Geometry: final body of the model. Coordinates: model frame, mm. A direction names the side the tool comes from. Round coordinates to 2 decimals unless told otherwise and drop trailing zeros. Order: outer loops, then holes, each group sorted by start corner. A loop starts at its lowest first (then second) coordinate and runs counter-clockwise, first axis right, second up. Notation, with made-up numbers: M 6,81 L 64,81 A17 ccw 64,96 Z; hole C 38.5,46.5 d1. An arc over 180 degrees is marked long. Return JSON: item names as keys, results as strings. Group by question number.
Q1. Cut plane B-B on x = 0. Output: boundary loops of the cut face in (y, z), and give its area (3 significant figures).
Q2. Cut plane A-A on y = 4.25. Output: boundary loops of the cut face in (x, z).
Q3. Access query for faces 1 (the face through (-1.5, 2.46, 0.07)), 2 (the face through (-1.74, 3.94, 0.99)), 3 (the face through (2, 8, 0)). Directions: +Z, -Z, +X, -X, +Y, -Y. A direction counts if a zero-diameter tool reaches every point of the face in a straight line with its end or side. Return the directions, or none.
Q4. Contact query for flat-ended pins moving along their axis: pin 1 (1.5 mm diameter, centred on x = 1, y = 10.5, fed in from -Z); pin 2 (1.8 mm diameter, centred on x = 0, z = 0, fed in from -Y); pin 3 (1.5 mm diameter, centred on y = 11.5, z = 1, fed in from +X). Output: stop coordinate, or through.
Q5. Mould query, pull axis Z, two halves, no side actions, for faces 4 (the face through (0, 16, 0)), 5 (the face through (0, 5, 0)), 6 (the face through (-1.5, 11.94, -0.07)). Classes: released by +Z, released by -Z, zero draft, split by the parting line, or undercut.
Q6. Ray query, probe 1 along Z at (x, y) = (0, 1.4); probe 2 along Y at (x, z) = (-1.4, 1.1); probe 3 along Y at (x, z) = (0.05, -0.5). Return the intervals inside material, ascending.
Q7. Cut plane C-C on z = 1. Output: boundary loops of the cut face in (x, y).
Q8. Cut plane D-D on y = 6. Output: boundary loops of the cut face in (x, z).
```python
from build123d import *

# Parameters (mm, degrees)
EXTRUDE_1_DEPTH     = 8
SKETCH_2_R          = 1.5
EXTRUDE_2_DEPTH     = 8
SKETCH_3_R          = 1.5
CUT_EXTRUDE_1_DEPTH = 5


with BuildPart() as part:
    # 草图1 → 凸台-拉伸1 (new body)
    with BuildSketch(Plane(origin=(0, 0, 0), x_dir=(1, 0, 0), z_dir=(0, 1, 0))):
        Polygon((-1.154700538, -2), (1.154700538, -2), (2.309401077, 0), (1.154700538, 2), (-1.154700538, 2), (-2.309401077, 0), align=None)
    extrude(amount=EXTRUDE_1_DEPTH)

    # 草图2 → 凸台-拉伸2 (add)
    with BuildSketch(Plane(origin=(0, 8, 0), x_dir=(1, 0, 0), z_dir=(0, 1, 0))):
        Circle(SKETCH_2_R)
    extrude(amount=EXTRUDE_2_DEPTH)

    # 草图3 → 切除-拉伸1 (cut)
    with BuildSketch(Plane.XZ):
        Circle(SKETCH_3_R)
    extrude(amount=-CUT_EXTRUDE_1_DEPTH, mode=Mode.SUBTRACT)


solid = part.part
```
Result sheet:
{
 "1": {"outline": "M 0,-2 L 8,-2 L 8,-1.5 L 16,-1.5 L 16,1.5 L 8,1.5 L 8,2 L 0,2 L 0,1.5 L 5,1.5 L 5,-1.5 L 0,-1.5 Z", "area": "41.0 mm²"},
 "2": {"outline": "M -2.31,0 L -1.15,-2 L 1.15,-2 L 2.31,0 L 1.15,2 L -1.15,2 Z; hole C 0,0 d3"},
 "3": {"face 1": "-Y", "face 2": "+Z, -X, +Y, -Y", "face 3": "+Y"},
 "4": {"pin 1": "stops at z = -1.48", "pin 2": "stops at y = 5", "pin 3": "stops at x = 1.48"},
 "5": {"face 4": "zero draft", "face 5": "undercut", "face 6": "split by the parting line"},
 "6": {"probe 1": "z = -2 to -1.5, 1.5 to 2", "probe 2": "y = 0 to 8", "probe 3": "y = 5 to 16"},
 "7": {"outline": "M -1.73,0 L -1.12,0 L -1.12,5 L 1.12,5 L 1.12,0 L 1.73,0 L 1.73,8 L 1.12,8 L 1.12,16 L -1.12,16 L -1.12,8 L -1.73,8 Z"},
 "8": {"outline": "M -2.31,0 L -1.15,-2 L 1.15,-2 L 2.31,0 L 1.15,2 L -1.15,2 Z"}
}
